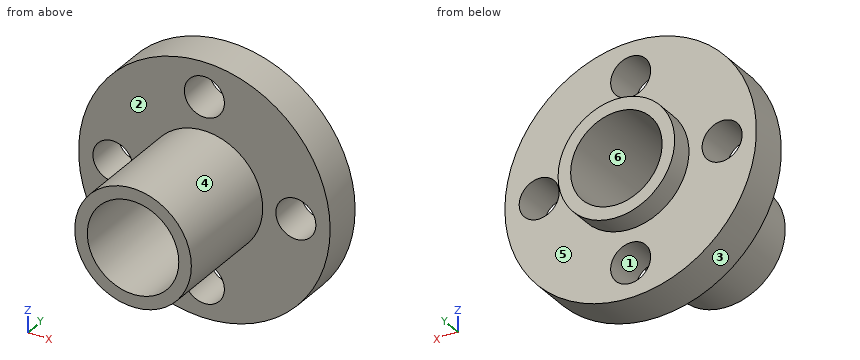
```python
from build123d import *

# Parameters (mm, degrees)
SKETCH_1_R          = 5.1
EXTRUDE_1_DEPTH     = 10
SKETCH_2_R          = 11
EXTRUDE_2_DEPTH     = 3.5
SKETCH_3_R          = 5.1
EXTRUDE_3_DEPTH     = 2
SKETCH_4_R          = 4
SKETCH_4_R_2        = 1.75
CUT_EXTRUDE_1_DEPTH = 16.5


with BuildPart() as part:
    # 草图1 → 凸台-拉伸1 (new body)
    with BuildSketch(Plane(origin=(0, 0, 0), x_dir=(1, 0, 0), z_dir=(0, 1, 0))):
        Circle(SKETCH_1_R)
    extrude(amount=EXTRUDE_1_DEPTH)

    # 草图2 → 凸台-拉伸2 (add)
    with BuildSketch(Plane(origin=(0, 10, 0), x_dir=(1, 0, 0), z_dir=(0, 1, 0))):
        Circle(SKETCH_2_R)
    extrude(amount=EXTRUDE_2_DEPTH)

    # 草图3 → 凸台-拉伸3 (add)
    with BuildSketch(Plane(origin=(0, 13.5, 0), x_dir=(1, 0, 0), z_dir=(0, 1, 0))):
        Circle(SKETCH_3_R)
    extrude(amount=EXTRUDE_3_DEPTH)

    # 草图4 → 切除-拉伸1 (cut, through all)
    with BuildSketch(Plane(origin=(0, 15.5, 0), x_dir=(1, 0, 0), z_dir=(0, 1, 0))):
        Circle(SKETCH_4_R)
        with Locations((-8, 0)):
            Circle(SKETCH_4_R_2)
        with Locations((0, -8)):
            Circle(SKETCH_4_R_2)
        with Locations((8, 0)):
            Circle(SKETCH_4_R_2)
        with Locations((0, 8)):
            Circle(SKETCH_4_R_2)
    extrude(amount=-CUT_EXTRUDE_1_DEPTH, mode=Mode.SUBTRACT)


solid = part.part
```
The listing builds one solid part. Answer for the finished solid, in the listing's coordinates (mm). Face numbers are marked on the shaded views. A direction names the side the tool comes from. Give positions to 0.01 mm unless a question says otherwise; leave off trailing zeros. Loops run counter-clockwise (first coordinate to the right, second up) from the corner with the lowest first, then second, coordinate; pieces in that order, holes last. Notation, with made-up numbers: (35.25, 59) - (42.25, 59) arc R28 cw to (42.25, 96) - close; hole circle Ø9 at (28, 25.25). An arc over 180 degrees is marked (long way). Return JSON: item names as keys, results as strings. Group by question number.
1. Find section C-C (z = 3.5). Write down the section's boundary in (x, y), then the cut area to 3 significant figures.
2. Straight lines are drawn through the part: line 1 (Z direction, x = 0, y = 10.9); line 2 (Z direction, x = -1, y = 12). For each, find the intervals that lie inside material, in ascending order. Write a range as [from, to].
3. Find section B-B (x = 0). Write down the section's boundary in (y, z).
4. Determine the mould class of the marked faces 1, 2 and 3 for opening direction Z: pulls with the +Z half, pulls with the -Z half, needs draft (parallel to the pull), parting line crosses it, or undercut.
5. Which of the six approach directions +Z, -Z, +X, -X, +Y, -Y give full straight-line access (tool end or side, diameter ignored) to the marked faces 4, 5 and 6?
6. Find section D-D (x = 7.25). Write down the section's boundary in (y, z), then the cut area to 3 significant figures.
7. Find section A-A (z = 0). Write down the section's boundary in (x, y).
8. Given pin 1 Ø5 at (x, z) = (8.5, 8) entering from -Y; pin 2 Ø3 at (x, z) = (0, -8) entering from -Y; pin 3 Ø2 at (y, z) = (8.5, -2) entering from +X; pin 4 Ø4 at (y, z) = (11, 8) entering from +X, each flat-ended and moving along its own axis, determine where each tip first touches the part or whether it passes through.
Verdict:
{
 "1": {"outline": "(-10.43, 10) - (-3.71, 10) - (-3.71, 0) - (-1.94, 0) - (-1.94, 15.5) - (-3.71, 15.5) - (-3.71, 13.5) - (-10.43, 13.5) - close; (1.94, 0) - (3.71, 0) - (3.71, 10) - (10.43, 10) - (10.43, 13.5) - (3.71, 13.5) - (3.71, 15.5) - (1.94, 15.5) - close", "area": "102 mm^2"},
 "2": {"line 1": "z = [-11, -9.75], [-6.25, -4], [4, 6.25], [9.75, 11]", "line 2": "z = [-10.95, -9.44], [-6.56, -3.87], [3.87, 6.56], [9.44, 10.95]"},
 "3": {"outline": "(0, -5.1) - (10, -5.1) - (10, -6.25) - (13.5, -6.25) - (13.5, -5.1) - (15.5, -5.1) - (15.5, -4) - (0, -4) - close; (0, 4) - (15.5, 4) - (15.5, 5.1) - (13.5, 5.1) - (13.5, 6.25) - (10, 6.25) - (10, 5.1) - (0, 5.1) - close; (10, -11) - (13.5, -11) - (13.5, -9.75) - (10, -9.75) - close; (10, 9.75) - (13.5, 9.75) - (13.5, 11) - (10, 11) - close"},
 "4": {"face 1": "undercut", "face 2": "needs draft", "face 3": "parting line crosses it"},
 "5": {"face 4": "-Y", "face 5": "+Y", "face 6": "+Y, -Y"},
 "6": {"outline": "(10, -8.27) - (13.5, -8.27) - (13.5, -1.58) - (10, -1.58) - close; (10, 1.58) - (13.5, 1.58) - (13.5, 8.27) - (10, 8.27) - close", "area": "46.8 mm^2"},
 "7": {"outline": "(-11, 10) - (-9.75, 10) - (-9.75, 13.5) - (-11, 13.5) - close; (-6.25, 10) - (-5.1, 10) - (-5.1, 0) - (-4, 0) - (-4, 15.5) - (-5.1, 15.5) - (-5.1, 13.5) - (-6.25, 13.5) - close; (4, 0) - (5.1, 0) - (5.1, 10) - (6.25, 10) - (6.25, 13.5) - (5.1, 13.5) - (5.1, 15.5) - (4, 15.5) - close; (9.75, 10) - (11, 10) - (11, 13.5) - (9.75, 13.5) - close"},
 "8": {"pin 1": "stops at y = 10", "pin 2": "passes through", "pin 3": "stops at x = 5", "pin 4": "stops at x = 9.22"}
}
